```python
from build123d import *

# Parameters (mm, degrees)
SKETCH1_W            = 89.72
SKETCH1_H            = 227
SKETCH1_R            = 2
HEAT_EXCHANGER_DEPTH = 0.1524
CONVECTION_FIN_DEPTH = 15.45166


with BuildPart() as part:
    # Sketch1 → Heat Exchanger (new body)
    with BuildSketch(Plane.XY):
        with Locations((-44.86, 0)):
            Rectangle(SKETCH1_W, SKETCH1_H)
        with Locations((-83.72, -56.6738)):
            Circle(SKETCH1_R, mode=Mode.SUBTRACT)
        with Locations((-83.72, 56.9786)):
            Circle(SKETCH1_R, mode=Mode.SUBTRACT)
    heat_exchanger = extrude(amount=HEAT_EXCHANGER_DEPTH)

    # Sketch3 → Convection Fin (add)
    with BuildSketch(Plane.XY):
        Polygon((0, -113.6524), (0, -113.5), (-89.72, -113.5), (-89.72, 113.5), (-89.8724, 113.5), (-89.8724, -113.6524), align=None)
    convection_fin = extrude(amount=CONVECTION_FIN_DEPTH)

    # Mirror1: Heat Exchanger, Convection Fin across plane
    add(heat_exchanger.mirror(Plane(origin=(0, 0, 0), x_dir=(0, 0, 1), z_dir=(1, 0, 0))))
    add(convection_fin.mirror(Plane(origin=(0, 0, 0), x_dir=(0, 0, 1), z_dir=(1, 0, 0))))


solid = part.part
```
For this review, take the finished solid that the model builds, in its own axes (mm). A direction names the side the tool comes from. Give positions to 0.01 mm unless a question says otherwise; leave off trailing zeros. Write each loop counter-clockwise with the first axis right and the second up, starting at its lowest first coordinate (ties: lowest second). Pieces come first, ordered by that corner, then holes. Notation, with made-up numbers: M 51,-13.5 L 94,-13.5 A22 cw 94,10.5 Z; hole C -6,28 d9. An arc over 180 degrees is marked long. Answer as a JSON object with one key per item and string values. Group by question number.
Item 1: Tool access review of faces 1 (the flat face through (1, -113.652, 8)), 2 (the flat face through (1, 2, 0.152)): name each direction out of +Z, -Z, +X, -X, +Y, -Y from which nothing blocks a thin tool from reaching the whole face with its end or side.
Item 2: Consider section C-C on x = -50.5. Write out the cut boundary in (y, z), plus the area to 3 significant figures.
Item 3: For pin 1 Ø5 at (x, y) = (62, -47) entering from +Z; pin 2 Ø3 at (x, z) = (32.5, 11) entering from +Y; pin 3 Ø1 at (x, y) = (33, -87) entering from -Z; pin 4 Ø3 at (x, y) = (83.72, -56.67) entering from +Z, all flat-tipped, find the tip position at first contact; note any pin that passes through.
Item 4: Consider section A-A on y = 33. Write out the cut boundary in (x, z), plus the area to 3 significant figures.
Item 5: Consider section B-B on z = 11.5. Write out the cut boundary in (x, y).
Item 6: For probe 1 along Y at (x, z) = (-83.72, 0.1); probe 2 along X at (y, z) = (-11, 8.75); probe 3 along Z at (x, y) = (-36, -39), list the stretches that pass through material, from the lowest coordinate up. Write a range as [from, to].
Item 7: Draft analysis for pull direction X (two halves, no side actions). For faces 3 (the flat face through (1, 2, 0)), 4 (the flat face through (89.72, -2, 8)), 5 (the flat face through (-89.872, 2, 8)), state which applies: +X half, -X half, draft (parallel to the pull), parting line (faces both ways), or undercut.
Check result:
{
 "1": {"face 1": "+Z, -Z, +X, -X, -Y", "face 2": "+Z, +Y"},
 "2": {"outline": "M -113.65,0 L 113.5,0 L 113.5,0.15 L -113.5,0.15 L -113.5,15.45 L -113.65,15.45 Z", "area": "36.9 mm^2"},
 "3": {"pin 1": "stops at z = 0.15", "pin 2": "stops at y = -113.5", "pin 3": "stops at z = 0", "pin 4": "passes through"},
 "4": {"outline": "M -89.87,0 L 89.87,0 L 89.87,15.45 L 89.72,15.45 L 89.72,0.15 L -89.72,0.15 L -89.72,15.45 L -89.87,15.45 Z", "area": "32.1 mm^2"},
 "5": {"outline": "M -89.87,-113.65 L 89.87,-113.65 L 89.87,113.5 L 89.72,113.5 L 89.72,-113.5 L -89.72,-113.5 L -89.72,113.5 L -89.87,113.5 Z"},
 "6": {"probe 1": "y = [-113.65, -58.67], [-54.67, 54.98], [58.98, 113.5]", "probe 2": "x = [-89.87, -89.72], [89.72, 89.87]", "probe 3": "z = [0, 0.15]"},
 "7": {"face 3": "draft", "face 4": "undercut", "face 5": "-X half"}
}
